```python
from build123d import *

# Parameters (mm, degrees)
BOSS_EXTRUDE1_DEPTH = 45
RIB1_REACH          = 327.464
SKETCH2_WALL_W      = 821.946192972
SKETCH2_WALL_H      = 20
SKETCH3_R           = 10
CUT_EXTRUDE1_DEPTH  = 313.929644864
FILLET1_R           = 40
SKETCH5_R           = 32
BOSS_EXTRUDE2_DEPTH = 40
SKETCH6_R           = 18.5
CUT_EXTRUDE2_DEPTH  = 320.005298403
RIB2_REACH          = 333.173
SKETCH7_WALL_W      = 701.683234458
SKETCH7_WALL_H      = 10
CIRPATTERN1_COUNT   = 4


with BuildPart() as part:
    # Sketch1 → Boss-Extrude1 (new, symmetric)
    with BuildSketch(Plane(origin=(0, 0, 0), x_dir=(0, 0, -1), z_dir=(1, 0, 0))):
        Polygon((0, 0), (129, 0), (244.5, 200.051868274), (227.179491924, 210.051868274), (117.452994616, 20), (0, 20), align=None)
    extrude(amount=BOSS_EXTRUDE1_DEPTH, both=True)

    # Sketch2 wall → Rib1 (add, up to next)
    with BuildSketch(Plane(origin=(0, 53.020201337, -77.790719439), x_dir=(0, 0.39073112849, -0.920504853452), z_dir=(0, 0.920504853452, 0.39073112849)), mode=Mode.PRIVATE) as rib1_sk1:
        Rectangle(SKETCH2_WALL_W, SKETCH2_WALL_H)
    rib1_tool1 = extrude(rib1_sk1.sketch, amount=-RIB1_REACH, mode=Mode.PRIVATE) - part.part
    add(rib1_tool1.solids().sort_by_distance((0, 53.020201337, -77.790719439))[0])

    # Sketch3 → Cut-Extrude1 (cut, through all)
    with BuildSketch(Plane(origin=(0, 20, 0), x_dir=(1, 0, 0), z_dir=(0, 1, 0))):
        with Locations(Location((-25, 20, 0), (0, 0, 270))):
            Circle(SKETCH3_R)
        with Locations(Location((-25, 89, 0), (0, 0, 270))):
            Circle(SKETCH3_R)
        with Locations(Location((25, 20, 0), (0, 0, 90))):
            Circle(SKETCH3_R)
        with Locations(Location((25, 89, 0), (0, 0, 90))):
            Circle(SKETCH3_R)
    extrude(amount=-CUT_EXTRUDE1_DEPTH, mode=Mode.SUBTRACT)

    # Fillet1
    fillet1_edges = [part.edges().sort_by_distance(p)[0] for p in [
        (45, 205.051868274, -235.839745962),
        (-45, 205.051868274, -235.839745962),
    ]]
    fillet(fillet1_edges, radius=FILLET1_R)

    # Sketch5 → Boss-Extrude2 (add)
    with BuildSketch(Plane(origin=(0, -45.858638544, -79.429491924), x_dir=(1, 0, 0), z_dir=(0, 0.49999999999999756, 0.86602540378444))):
        with Locations(Location((0, 250.5, 0), (0, 0, 90))):
            Circle(SKETCH5_R)
    extrude(amount=BOSS_EXTRUDE2_DEPTH)

    # Sketch6 → Cut-Extrude2 (cut, through all)
    with BuildSketch(Plane(origin=(0, -25.858638544, -44.788475773), x_dir=(1, 0, 0), z_dir=(0, 0.49999999999999756, 0.86602540378444))):
        with Locations(Location((0, 250.5, 0), (0, 0, 270))):
            Circle(SKETCH6_R)
    extrude(amount=-CUT_EXTRUDE2_DEPTH, mode=Mode.SUBTRACT)

    # Sketch7 wall → Rib2 (add, up to next)
    with BuildSketch(Plane(origin=(0, 213.172703149, -208.774047358), x_dir=(0, -0.16717425612, -0.985927364511), z_dir=(0, 0.985927364511, -0.16717425612)), mode=Mode.PRIVATE) as rib2_sk1:
        Rectangle(SKETCH7_WALL_W, SKETCH7_WALL_H)
    rib2_tool1 = extrude(rib2_sk1.sketch, amount=-RIB2_REACH, mode=Mode.PRIVATE) - part.part
    rib2 = rib2_tool1.solids().sort_by_distance((0, 213.172703149, -208.774047358))[0]
    add(rib2)

    # CirPattern1: Rib2 ×4 about axis
    cirpattern1_axis = Axis((0, 216.939363648, -125.25), (0, 0.49999999999999745, 0.8660254037844402))
    for i in range(1, CIRPATTERN1_COUNT):
        add(rib2.rotate(cirpattern1_axis, i * 360 / CIRPATTERN1_COUNT))


solid = part.part
```
Geometry: final body of the model. Coordinates: model frame, mm. A direction names the side the tool comes from. Round coordinates to 2 decimals unless told otherwise and drop trailing zeros. Order: outer loops, then holes, each group sorted by start corner. A loop starts at its lowest first (then second) coordinate and runs counter-clockwise, first axis right, second up. Notation, with made-up numbers: (22, -1) - (63, -1) arc R17 ccw to (63, 29) - close; hole circle Ø4 at (-8.75, 9.5). An arc over 180 degrees is marked (long way). Use CSV: the item, a comma, the result in double quotes. Start each with the question number.
Q1. Section query B-B (z = -20). Return loops of the section in (x, y), and give its area (3 significant figures).
Q2. Mould query, pull axis Y, two halves, no side actions, for faces 4 (the face through (33.6, 194.7, -229.7)), 5 (the face through (0.63, 94.4, -160.41)), 6 (the face through (22, 10.14, -29.54)). Classes: +Y half, -Y half, draft (parallel to the pull), parting line (faces both ways), or undercut.
Q3. Section query C-C (y = 76.5). Return loops of the section in (x, z).
Q4. Section query A-A (x = -28). Return loops of the section in (y, z), and give its area (3 significant figures).
Q5. Material intervals for line 1 along X through (y, z) = (5.75, -20); line 2 along Y through (x, z) = (-7, -185); line 3 along X through (y, z) = (51, -103), sorted ascending. Write a range as from..to.
Q6. Section query D-D (z = -142). Return loops of the section in (x, y), and give its area (3 significant figures).
Q7. First-contact query: pin 1 (17.5 mm diameter, centred on x = 34.5, z = -36, fed in from +Y); pin 2 (9 mm diameter, centred on y = 148, z = -180.5, fed in from +X); pin 3 (4 mm diameter, centred on x = 19.5, y = 167.5, fed in from +Z). Flat tips, straight axial feed; report the tip coordinate or a pass-through.
Q8. Access query for faces 1 (the face through (25.28, 192.974, -217.319)), 2 (the face through (10, 41, -82)), 3 (the face through (-36.51, 181.96, -195.84)). Directions: +Z, -Z, +X, -X, +Y, -Y. A direction counts if a zero-diameter tool reaches every point of the face in a straight line with its end or side. Return the directions, or none.
Result set:
1,outline,"(-45, 0) - (-35, 0) - (-35, 20) - (-45, 20) - close; (-15, 0) - (15, 0) - (15, 20) - (10, 20) - (10, 28.49) - (-10, 28.49) - (-10, 20) - (-15, 20) - close; (35, 0) - (45, 0) - (45, 20) - (35, 20) - close"
1,area,"1,170 mm2"
2,face 4,"+Y half"
2,face 5,"undercut"
2,face 6,"draft"
3,outline,"(-45, -173.17) - (45, -173.17) - (45, -150.07) - (10, -150.07) - (10, -133.11) - (-10, -133.11) - (-10, -150.07) - (-45, -150.07) - close"
4,outline,"(0, -129) - (193.75, -240.86) - (203.75, -223.54) - (184.5, -212.43) - (204.5, -177.78) - (177.66, -162.29) - (157.66, -196.93) - (20, -117.45) - (20, -98.54) - (0, -98.54) - close; (0, -79.46) - (20, -79.46) - (20, -29.54) - (0, -29.54) - close; (0, -10.46) - (20, -10.46) - (20, 0) - (0, 0) - close"
4,area,"7,300 mm2"
5,line 1,"x = -45..-35, -15..15, 35..45"
5,line 2,"y = 96.99..136.99, 146.39..162.67, 202.22..216.99"
5,line 3,"x = -10..10"
6,outline,"(-45, 22.52) - (45, 22.52) - (45, 62.52) - (10, 62.52) - (10, 80.28) - (-10, 80.28) - (-10, 62.52) - (-45, 62.52) - close"
6,area,"3,960 mm2"
7,pin 1,"stops at y = 20"
7,pin 2,"stops at x = 16.23"
7,pin 3,"stops at z = -156.66"
8,face 1,"+X, +Y"
8,face 2,"+Z, +X, +Y"
8,face 3,"-X, +Y"
